Geometry check sheet. Reference: drawing and pictorial views, mm from the part's lowest x, y, z. Give positions to 0.01 mm unless a question says otherwise; leave off trailing zeros. Order: outer loops, then holes, each group sorted by start corner. A loop starts at its lowest first (then second) coordinate and runs counter-clockwise, first axis right, second up. Notation, with made-up numbers: (57.5, -7) - (104.5, -7) arc R29 ccw to (104.5, 13) - close; hole circle Ø10 at (45, -20). An arc over 180 degrees is marked (long way). Answer as a JSON object with one key per item and string values.
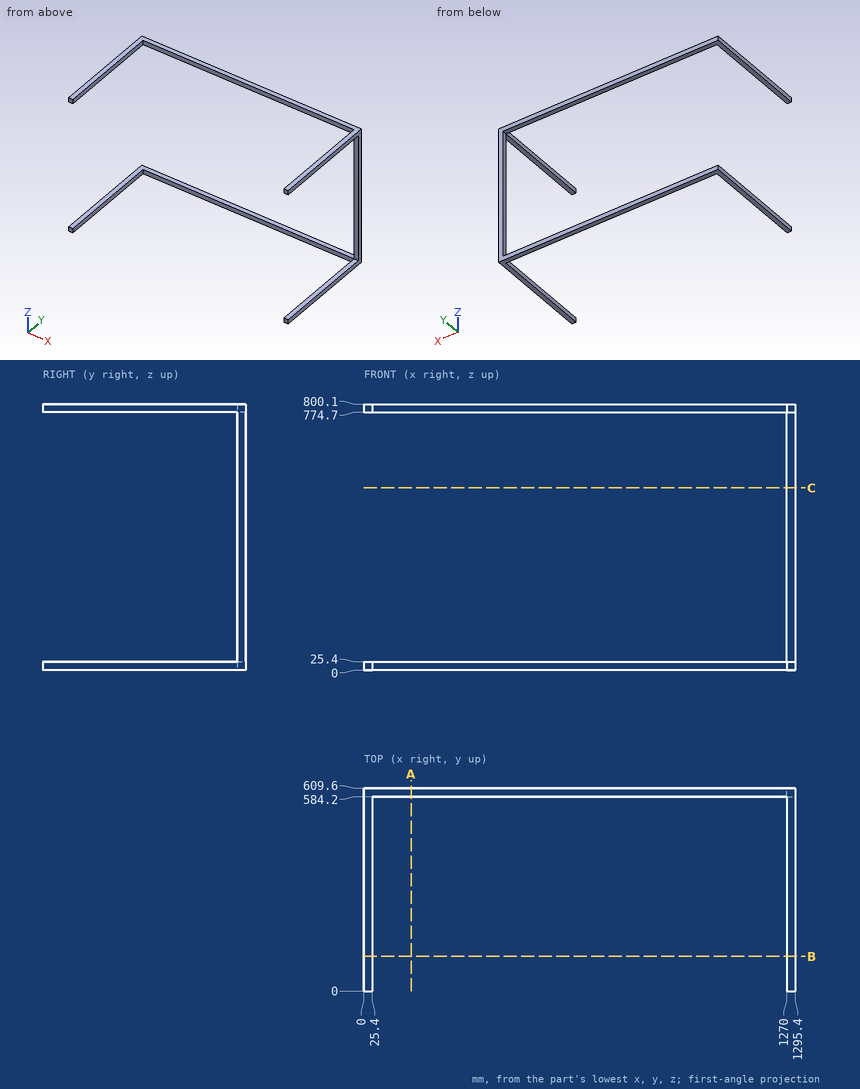
(1) Gauge pin test, flat ends, axial feed: pin 1 Ø7.5 at (x, y) = (1283, 280) entering from -Z; pin 2 Ø7.5 at (x, z) = (630, 786) entering from -Y. Record the tip position at first contact, or that the pin passes through.
Computed values:
{"pin 1": "stops at z = 0", "pin 2": "stops at y = 584.2"}
(2) Section check C-C (z = 548). Record the cut outline in (x, y).
Computed values:
{"outline": "(1270, 584.2) - (1295.4, 584.2) - (1295.4, 609.6) - (1270, 609.6) - close"}
(3) Section check A-A (x = 142). Record the cut outline in (y, z), then the cut area to 3 significant figures.
Computed values:
{"outline": "(584.2, 0) - (609.6, 0) - (609.6, 25.4) - (584.2, 25.4) - close; (584.2, 774.7) - (609.6, 774.7) - (609.6, 800.1) - (584.2, 800.1) - close", "area": "1,290 mm²"}
(4) Section check B-B (y = 104.5). Record the cut outline in (x, z).
Computed values:
{"outline": "(0, 0) - (25.4, 0) - (25.4, 25.4) - (0, 25.4) - close; (0, 774.7) - (25.4, 774.7) - (25.4, 800.1) - (0, 800.1) - close; (1270, 0) - (1295.4, 0) - (1295.4, 25.4) - (1270, 25.4) - close; (1270, 774.7) - (1295.4, 774.7) - (1295.4, 800.1) - (1270, 800.1) - close"}
